Part print with two shaded views. Sizes in mm from the minimum x, y, z corner. Coordinates: 2 decimals unless noted, no trailing zeros. Loops run counter-clockwise (first coordinate to the right, second up) from the corner with the lowest first, then second, coordinate; pieces in that order, holes last.
(1) Flat gauge pins, fed straight in: P1, Ø3, axis at x = 11, y = 39, coming from the +Z side; P2, Ø1.5, axis at x = 34, z = 2.5, coming from the +Y side. Where does each tip first touch, or does it go through?
(2) Slice it at B-B (x = 38). Give the number of separate pieces and of enclosed holes in the cut face, and give its area (3 significant figures).
(3) Slice it at C-C (z = 2.5). Give the cut face in (x, y), and give its area (3 significant figures).
(4) Slice it at A-A (y = 58). Give the cut face in (x, z).
(5) Wall check: L1, parallel to Y at x = 38, z = 0.2; L2, parallel to Y at x = 11.5, z = 1.7; L3, parallel to X at y = 47.5, z = 0.8. Give the ranges that are in metal, low to high.
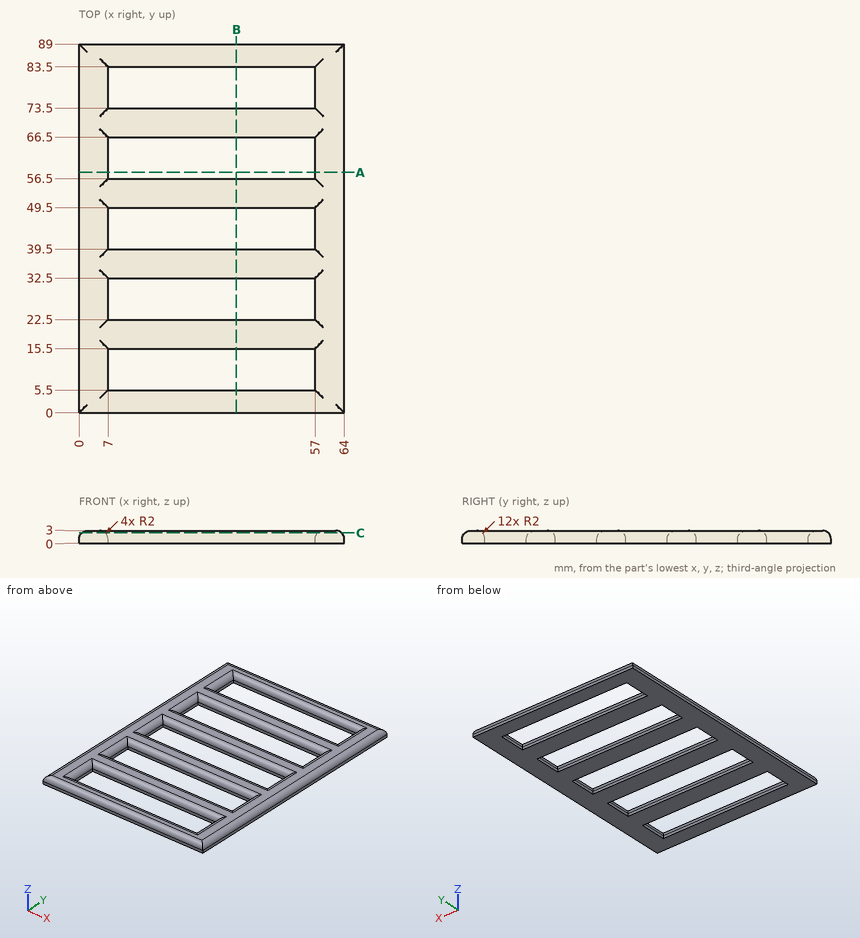
Response values:
1. P1: stops at z = 3
1. P2: stops at y = 88.85
2. separate pieces: 6
2. enclosed holes: 0
2. area: 107 mm2
3. outline: (0.68, 0.68) - (63.32, 0.68) - (63.32, 88.32) - (0.68, 88.32) - close; hole (6.32, 4.82) - (57.68, 4.82) - (57.68, 16.18) - (6.32, 16.18) - close; hole (6.32, 21.82) - (57.68, 21.82) - (57.68, 33.18) - (6.32, 33.18) - close; hole (6.32, 38.82) - (57.68, 38.82) - (57.68, 50.18) - (6.32, 50.18) - close; hole (6.32, 55.82) - (57.68, 55.82) - (57.68, 67.18) - (6.32, 67.18) - close; hole (6.32, 72.82) - (57.68, 72.82) - (57.68, 84.18) - (6.32, 84.18) - close
3. area: 2,580 mm2
4. outline: (0, 0) - (7, 0) - (7, 1) arc R2 ccw to (5, 3) - (2, 3) arc R2 ccw to (0, 1) - close; (57, 0) - (64, 0) - (64, 1) arc R2 ccw to (62, 3) - (59, 3) arc R2 ccw to (57, 1) - close
5. L1: y = 0 to 5.5, 15.5 to 22.5, 32.5 to 39.5, 49.5 to 56.5, 66.5 to 73.5, 83.5 to 89
5. L2: y = 0.13 to 5.37, 15.63 to 22.37, 32.63 to 39.37, 49.63 to 56.37, 66.63 to 73.37, 83.63 to 88.87
5. L3: x = 0 to 7, 57 to 64
